```python
from build123d import *

# Parameters (mm, degrees)
SKETCH1_W               = 8
SKETCH1_H               = 8
BOSS_EXTRUDE1_DEPTH     = 3
CUT_EXTRUDE1_DEPTH      = 12.704699911
CUT_EXTRUDE1_DEPTH_BACK = 12.704699911
CUT_EXTRUDE2_DEPTH      = 11
SKETCH4_R               = 1.75
CUT_EXTRUDE3_DEPTH      = 0.4
SKETCH5_W               = 8
SKETCH5_H               = 1
BOSS_EXTRUDE2_DEPTH     = 2
FILLET1_R               = 4
CUT_EXTRUDE4_DEPTH      = 0.4
CUT_EXTRUDE5_DEPTH      = 0.5


with BuildPart() as part:
    # Sketch1 → Boss-Extrude1 (new body)
    with BuildSketch(Plane(origin=(0, 0, 0), x_dir=(1, 0, 0), z_dir=(0, 1, 0))):
        with Locations((4, 4)):
            Rectangle(SKETCH1_W, SKETCH1_H)
    extrude(amount=BOSS_EXTRUDE1_DEPTH)

    # Sketch2 → Cut-Extrude1 (cut, two sides: drawn at the far end of the back side and taken through both)
    with BuildSketch(Plane.XY.offset(-CUT_EXTRUDE1_DEPTH_BACK)):
        Polygon((0, 0), (0.6, 3), (0, 3), align=None)
        Polygon((8, 0), (7.4, 3), (8, 3), align=None)
    extrude(amount=CUT_EXTRUDE1_DEPTH + CUT_EXTRUDE1_DEPTH_BACK, mode=Mode.SUBTRACT)

    # Sketch3 → Cut-Extrude2 (cut)
    with BuildSketch(Plane(origin=(0, 0, 0), x_dir=(0, 0, -1), z_dir=(1, 0, 0))):
        Polygon((0, 0), (0.6, 3), (0, 3), align=None)
        Polygon((8, 3), (7.4, 3), (8, 0), align=None)
    extrude(amount=CUT_EXTRUDE2_DEPTH, mode=Mode.SUBTRACT)

    # Sketch4 → Cut-Extrude3 (cut)
    with BuildSketch(Plane.XZ):
        with Locations(Location((4, -3.75, 0), (0, 0, 270))):
            Circle(SKETCH4_R)
    extrude(amount=-CUT_EXTRUDE3_DEPTH, mode=Mode.SUBTRACT)

    # Sketch5 → Boss-Extrude2 (add)
    with BuildSketch(Plane.XZ):
        with Locations((4, -7.5)):
            Rectangle(SKETCH5_W, SKETCH5_H)
    extrude(amount=BOSS_EXTRUDE2_DEPTH)

    # Fillet1
    # the kernel refuses this fillet: 4 mm, written as the material it takes off along each edge
    with BuildSketch(Plane(origin=(8, -2, -16.660254038), x_dir=(0, 1, 0), z_dir=(0, 0, 1)), Plane(origin=(0, -2, 1.660254038), x_dir=(0, 1, 0), z_dir=(0, 0, -1))) as fillet1_piece_1:
        with BuildLine():
            CenterArc((4, 3.464101615), FILLET1_R, 180, 60)
            Line((0, 3.464101615), (-0.08, 3.464101615))
            Line((-0.08, 3.464101615), (-0.08, 0))
            Line((-0.08, 0), (0, -0.08))
            ThreePointArc((0, -0.08), (1, -0.08), (1.96, -0.069282032))
            Line((1.96, -0.069282032), (2, 0))
        make_face()
    extrude(amount=18.320508076, mode=Mode.SUBTRACT)

    # Sketch6 → Cut-Extrude4 (cut)
    with BuildSketch(Plane(origin=(0, 3, 0), x_dir=(1, 0, 0), z_dir=(0, 1, 0))):
        with BuildLine():
            Line((4.478635236, 6.002856352), (5.247866005, 6.002856352))
            Line((5.247866005, 6.002856352), (5.247866005, 3.481221736))
            add(Edge.make_bspline(
                [(5.247866005, 3.481221736), (5.247522255, 3.441153869), (5.246855206, 3.363401883), (5.242756502, 3.250390465), (5.236658321, 3.14454193), (5.227277222, 3.045871471), (5.21405872, 2.954592388), (5.200049867, 2.869976575), (5.183041427, 2.792451692), (5.167800036, 2.743951306), (5.160526262, 2.72080507)],
                knots=[0, 0, 0, 0, 1.251619961, 2.428777588, 3.532126049, 4.56323557, 5.523704531, 6.412540087, 7.242403515, 8, 8, 8, 8], degree=3))
            add(Edge.make_bspline(
                [(5.160526262, 2.72080507), (5.150361081, 2.692282601), (5.130243602, 2.635834988), (5.091141653, 2.555314881), (5.046176431, 2.479084315), (4.995474484, 2.406812938), (4.939514717, 2.338210987), (4.876399077, 2.275086649), (4.8083478, 2.215238098), (4.733446681, 2.161145289), (4.653580791, 2.110709794), (4.566475051, 2.068688963), (4.473843299, 2.032340387), (4.374908104, 2.002816628), (4.269640778, 1.979716073), (4.158311001, 1.962901894), (4.040770466, 1.95334773), (3.960490164, 1.952175274), (3.919340364, 1.9515743)],
                knots=[0, 0, 0, 0, 0.925533072, 1.831683394, 2.73255258, 3.630007683, 4.529542467, 5.436465751, 6.357118906, 7.298274949, 8.259461937, 9.242242071, 10.251058183, 11.300341426, 12.396409345, 13.544807631, 14.74152597, 16, 16, 16, 16], degree=3))
            add(Edge.make_bspline(
                [(3.919340364, 1.9515743), (3.871225528, 1.952737211), (3.777685944, 1.954998015), (3.641661475, 1.97000769), (3.514100564, 1.996260242), (3.395387048, 2.034179675), (3.284307874, 2.08131717), (3.182206561, 2.140114726), (3.088540477, 2.209392701), (3.003918711, 2.289363431), (2.928299433, 2.379218215), (2.863026475, 2.479745415), (2.80762712, 2.589893743), (2.762984692, 2.710161506), (2.727739397, 2.839972913), (2.702317462, 2.979601288), (2.687147894, 3.129126134), (2.684913172, 3.2319872), (2.683763441, 3.284907634)],
                knots=[0, 0, 0, 0, 1.114068574, 2.165849827, 3.164101702, 4.124467949, 5.046988974, 5.952942428, 6.846011651, 7.738523925, 8.642829306, 9.558838605, 10.50752403, 11.491963144, 12.524197802, 13.618364352, 14.774685164, 16, 16, 16, 16], degree=3))
            Line((2.683763441, 3.284907634), (3.45299421, 3.336189685))
            add(Edge.make_bspline(
                [(3.45299421, 3.336189685), (3.454375767, 3.307862598), (3.45702498, 3.25354382), (3.464380935, 3.175240866), (3.473682687, 3.103271277), (3.485853837, 3.037851064), (3.498960823, 2.978427444), (3.515987002, 2.926169857), (3.533886556, 2.879240769), (3.549608387, 2.851783511), (3.557160877, 2.838593531)],
                knots=[0, 0, 0, 0, 1.326609226, 2.543847584, 3.678365909, 4.719972403, 5.656527627, 6.521948534, 7.28997025, 8, 8, 8, 8], degree=3))
            add(Edge.make_bspline(
                [(3.557160877, 2.838593531), (3.56872297, 2.821148121), (3.59147861, 2.786813382), (3.632990929, 2.742071605), (3.677558537, 2.702955843), (3.727619554, 2.672203009), (3.781780527, 2.648016829), (3.840448037, 2.63044225), (3.903460331, 2.619785853), (3.946808463, 2.61876437), (3.969019851, 2.618240967)],
                knots=[0, 0, 0, 0, 1.023658308, 2.014687051, 2.979722519, 3.920049697, 4.880550909, 5.878122304, 6.912759386, 8, 8, 8, 8], degree=3))
            add(Edge.make_bspline(
                [(3.969019851, 2.618240967), (3.991477248, 2.618659453), (4.034647527, 2.619463917), (4.09686091, 2.626779219), (4.154063033, 2.638632824), (4.206285054, 2.655294856), (4.253703868, 2.676924623), (4.295268393, 2.704596166), (4.33276969, 2.735732915), (4.36516489, 2.773188264), (4.392766236, 2.818318957), (4.415812105, 2.873248962), (4.43563784, 2.938204221), (4.450960178, 3.01367855), (4.464002509, 3.098949399), (4.472183692, 3.194770716), (4.478064386, 3.300859295), (4.478439634, 3.37517575), (4.478635236, 3.413914044)],
                knots=[0, 0, 0, 0, 0.980314827, 1.884477813, 2.730827652, 3.527503874, 4.27366112, 4.998269146, 5.70163477, 6.396145331, 7.150281155, 8.001758491, 8.990432449, 10.111292654, 11.361572691, 12.75538406, 14.308707205, 16, 16, 16, 16], degree=3))
            Line((4.478635236, 3.413914044), (4.478635236, 6.002856352))
        make_face()
    extrude(amount=-CUT_EXTRUDE4_DEPTH, mode=Mode.SUBTRACT)

    # Sketch7 → Cut-Extrude5 (cut)
    with BuildSketch(Plane(origin=(0, 3, 0), x_dir=(1, 0, 0), z_dir=(0, 1, 0))):
        Polygon((6.21271865, 2.977310221), (6.502782752, 2.977310221), (6.989962239, 0.977310221), (6.700298778, 0.977310221), align=None)
    extrude(amount=-CUT_EXTRUDE5_DEPTH, mode=Mode.SUBTRACT)


solid = part.part
```
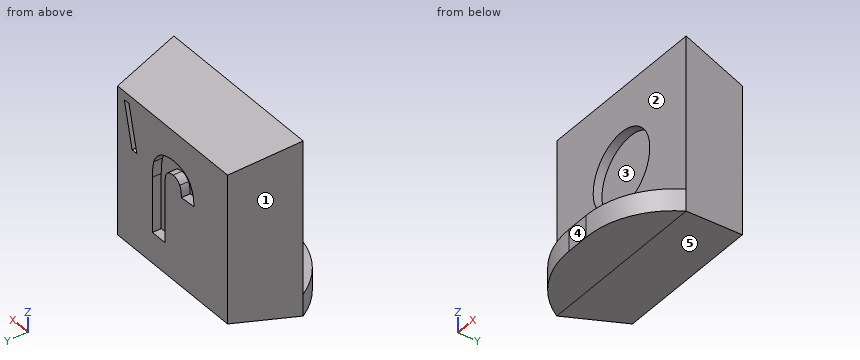
Source: CAD feature listing. Evaluate the final solid. Frame: model axes, mm. Face numbers are marked on the shaded views. A direction names the side the tool comes from. Round coordinates to 2 decimals unless told otherwise and drop trailing zeros. Loops run counter-clockwise (first coordinate to the right, second up) from the corner with the lowest first, then second, coordinate; pieces in that order, holes last. Notation, with made-up numbers: M -17.5,24 L 8.5,24 A26 cw 8.5,49 Z; hole C 38,56.25 d7. An arc over 180 degrees is marked long. Use a Markdown table: item, result. Add a question column.
1. Contact query for flat-ended pins moving along their axis: P1, Ø3, axis at y = 2, z = -2, coming from the -X side; P2, Ø3, axis at x = 4, z = -3, coming from the -Y side. Output: stop coordinate, or through.
2. Mould query, pull axis Z, two halves, no side actions, for the marked faces 3, 4 and 5. Classes: pulls with the +Z half, pulls with the -Z half, needs draft (parallel to the pull), parting line crosses it, or undercut.
3. Section query A-A on z = -3.75. Return the cut outline in (x, y), then the cut area to 3 significant figures.
4. Line query: line 1 (Y direction, x = 7, z = -6); line 2 (X direction, y = 0.25, z = -3.75); line 3 (X direction, y = 0.1, z = -3.75). Output: solid intervals per line, ascending.
5. Section query D-D on z = -7.25. Return the cut outline in (x, y).
6. Section query C-C on x = 5.5. Return the cut outline in (y, z).
7. Section query B-B on y = 1.3. Return the cut outline in (x, z), then the cut area to 3 significant figures.
8. Reachability of the marked faces 1 and 2 from +Z, -Z, +X, -X, +Y, -Y: full face, straight path, thin tool, end or side. Return the list, or none.
Reported:
| question | item | result |
|---|---|---|
| 1 | P1 | stops at x = 0.1 |
| 1 | P2 | stops at y = 0 |
| 2 | face 3 | undercut |
| 2 | face 4 | needs draft |
| 2 | face 5 | pulls with the -Z half |
| 3 | outline | M 0,0 L 2.25,0 L 2.25,0.4 L 5.75,0.4 L 5.75,0 L 8,0 L 7.4,3 L 5.25,3 L 5.25,2.6 L 4.48,2.6 L 4.48,3 L 0.6,3 Z |
| 3 | area | 20.5 mm² |
| 4 | line 1 | y = 0 to 3 |
| 4 | line 2 | x = 0.05 to 2.25, 5.75 to 7.95 |
| 4 | line 3 | x = 0.02 to 2.25, 5.75 to 7.98 |
| 5 | outline | M 0,0 A4 ccw 3.46,-2 L 4.54,-2 A4 ccw 8,0 L 7.4,3 L 0.6,3 Z |
| 6 | outline | M -1.88,-8 L 0,-8 L 3,-7.4 L 3,-0.6 L 0,0 L 0,-2.85 L 0.4,-2.85 L 0.4,-4.65 L 0,-4.65 L 0,-7 L -1.88,-7 Z |
| 7 | outline | M 0.26,-7.74 L 7.74,-7.74 L 7.74,-0.26 L 0.26,-0.26 Z |
| 7 | area | 56.0 mm² |
| 8 | face 1 | +Z, -Z, -X, +Y |
| 8 | face 2 | +Z, +X, -X, -Y |
